```python
from build123d import *

# Parameters (mm, degrees)
SKETCH_1_R           = 3.1
EXTRUDE_1_DEPTH      = 6
SKETCH_2_R           = 3.1
CUT_EXTRUDE_6_DEPTH  = 2
SKETCH_4_R           = 1.5
CUT_EXTRUDE_7_DEPTH  = 118.034622889
CUT_EXTRUDE_8_REACH  = 119.12
SKETCH_5_W           = 7
SKETCH_5_H           = 21.556656584
SKETCH_5_W_2         = 5.195776916
SKETCH_5_R           = 4
SKETCH_5_W_3         = 8.137387099
SKETCH_5_H_2         = 20
SKETCH_5_W_4         = 10
SKETCH_6_R           = 3.1
CUT_EXTRUDE_9_DEPTH  = 2
SKETCH_7_R           = 1.6
CUT_EXTRUDE_10_DEPTH = 118.034622889
SKETCH_8_R           = 1.5
CUT_EXTRUDE_11_DEPTH = 118.120036521
SKETCH_9_W           = 120
SKETCH_9_H           = 5
CUT_EXTRUDE_12_DEPTH = 2
CHAMFER_1_SIZE       = 2
SKETCH_10_W          = 120
SKETCH_10_H          = 4
EXTRUDE_2_DEPTH      = 2


with BuildPart() as part:
    # 草图1 → 凸台-拉伸1 (new body)
    with BuildSketch(Plane.XY):
        with BuildLine():
            Line((53.211823486, 15.105307707), (98.846336292, -57.534028788))
            Line((98.846336292, -57.534028788), (98.846336292, -62.534028788))
            Line((98.846336292, -62.534028788), (-21.153663708, -62.534028788))
            Line((-21.153663708, -62.534028788), (-21.153663708, -57.534028788))
            Line((-21.153663708, -57.534028788), (18.804405563, 14.198660069))
            ThreePointArc((18.804405563, 14.198660069), (35.749695352, 24.459031414), (53.211823486, 15.105307707))
        make_face()
        with Locations((36.276519563, 4.465971212)):
            Circle(SKETCH_1_R, mode=Mode.SUBTRACT)
    extrude(amount=EXTRUDE_1_DEPTH)

    # 草图2 → 切除-拉伸6 (cut)
    with BuildSketch(Plane.XY.offset(6)):
        with Locations((29.276519563, 11.465971212)):
            Circle(SKETCH_2_R)
        with Locations(Location((43.276519563, 11.465971212, 0), (0, 0, 180))):
            Circle(SKETCH_2_R)
        with Locations((43.276519563, -2.534028788)):
            Circle(SKETCH_2_R)
        with Locations(Location((29.276519563, -2.534028788, 0), (0, 0, 180))):
            Circle(SKETCH_2_R)
    extrude(amount=-CUT_EXTRUDE_6_DEPTH, mode=Mode.SUBTRACT)

    # 草图4 → 切除-拉伸7 (cut, through all)
    with BuildSketch(Plane.XY.offset(4)):
        with Locations((43.276519563, 11.465971212)):
            Circle(SKETCH_4_R)
        with Locations((43.276519563, -2.534028788)):
            Circle(SKETCH_4_R)
        with Locations((29.276519563, -2.534028788)):
            Circle(SKETCH_4_R)
        with Locations((29.276519563, 11.465971212)):
            Circle(SKETCH_4_R)
    extrude(amount=-CUT_EXTRUDE_7_DEPTH, mode=Mode.SUBTRACT)

    # 草图5 → 切除-拉伸8 (cut, up to next)
    with BuildSketch(Plane.XY.offset(6), mode=Mode.PRIVATE) as cut_extrude_8_sk1:
        with Locations((21.160819148, -19.755700496)):
            Rectangle(SKETCH_5_W, SKETCH_5_H)
    cut_extrude_8_tool1 = extrude(cut_extrude_8_sk1.sketch, amount=-CUT_EXTRUDE_8_REACH, mode=Mode.PRIVATE) & part.part
    # 草图5 → 切除-拉伸8 (cut, up to next)
    with BuildSketch(Plane.XY.offset(6), mode=Mode.PRIVATE) as cut_extrude_8_sk2:
        with Locations((31.160819148, -19.755700496)):
            Rectangle(SKETCH_5_W, SKETCH_5_H)
    cut_extrude_8_tool2 = extrude(cut_extrude_8_sk2.sketch, amount=-CUT_EXTRUDE_8_REACH, mode=Mode.PRIVATE) & part.part
    # 草图5 → 切除-拉伸8 (cut, up to next)
    with BuildSketch(Plane.XY.offset(6), mode=Mode.PRIVATE) as cut_extrude_8_sk3:
        with Locations((41.160819148, -19.755700496)):
            Rectangle(SKETCH_5_W, SKETCH_5_H)
    cut_extrude_8_tool3 = extrude(cut_extrude_8_sk3.sketch, amount=-CUT_EXTRUDE_8_REACH, mode=Mode.PRIVATE) & part.part
    # 草图5 → 切除-拉伸8 (cut, up to next)
    with BuildSketch(Plane.XY.offset(6), mode=Mode.PRIVATE) as cut_extrude_8_sk4:
        with Locations((51.160819148, -19.755700496)):
            Rectangle(SKETCH_5_W, SKETCH_5_H)
    cut_extrude_8_tool4 = extrude(cut_extrude_8_sk4.sketch, amount=-CUT_EXTRUDE_8_REACH, mode=Mode.PRIVATE) & part.part
    # 草图5 → 切除-拉伸8 (cut, up to next)
    with BuildSketch(Plane.XY.offset(6), mode=Mode.PRIVATE) as cut_extrude_8_sk5:
        with Locations((60.258707606, -19.755700496)):
            Rectangle(SKETCH_5_W_2, SKETCH_5_H)
    cut_extrude_8_tool5 = extrude(cut_extrude_8_sk5.sketch, amount=-CUT_EXTRUDE_8_REACH, mode=Mode.PRIVATE) & part.part
    # 草图5 → 切除-拉伸8 (cut, up to next)
    with BuildSketch(Plane.XY.offset(6), mode=Mode.PRIVATE) as cut_extrude_8_sk6:
        with Locations((14.988200827, -44.534028788)):
            Circle(SKETCH_5_R)
    cut_extrude_8_tool6 = extrude(cut_extrude_8_sk6.sketch, amount=-CUT_EXTRUDE_8_REACH, mode=Mode.PRIVATE) & part.part
    # 草图5 → 切除-拉伸8 (cut, up to next)
    with BuildSketch(Plane.XY.offset(6), mode=Mode.PRIVATE) as cut_extrude_8_sk7:
        with Locations((44.988200827, -44.534028788)):
            Circle(SKETCH_5_R)
    cut_extrude_8_tool7 = extrude(cut_extrude_8_sk7.sketch, amount=-CUT_EXTRUDE_8_REACH, mode=Mode.PRIVATE) & part.part
    # 草图5 → 切除-拉伸8 (cut, up to next)
    with BuildSketch(Plane.XY.offset(6), mode=Mode.PRIVATE) as cut_extrude_8_sk8:
        with Locations((74.988200827, -44.534028788)):
            Circle(SKETCH_5_R)
    cut_extrude_8_tool8 = extrude(cut_extrude_8_sk8.sketch, amount=-CUT_EXTRUDE_8_REACH, mode=Mode.PRIVATE) & part.part
    # 草图5 → 切除-拉伸8 (cut, up to next)
    with BuildSketch(Plane.XY.offset(6), mode=Mode.PRIVATE) as cut_extrude_8_sk9:
        with Locations((1.433627507, -44.534028788)):
            Rectangle(SKETCH_5_W_3, SKETCH_5_H_2)
    cut_extrude_8_tool9 = extrude(cut_extrude_8_sk9.sketch, amount=-CUT_EXTRUDE_8_REACH, mode=Mode.PRIVATE) & part.part
    # 草图5 → 切除-拉伸8 (cut, up to next)
    with BuildSketch(Plane.XY.offset(6), mode=Mode.PRIVATE) as cut_extrude_8_sk10:
        with Locations((30.502321056, -44.534028788)):
            Rectangle(SKETCH_5_W_4, SKETCH_5_H_2)
    cut_extrude_8_tool10 = extrude(cut_extrude_8_sk10.sketch, amount=-CUT_EXTRUDE_8_REACH, mode=Mode.PRIVATE) & part.part
    # 草图5 → 切除-拉伸8 (cut, up to next)
    with BuildSketch(Plane.XY.offset(6), mode=Mode.PRIVATE) as cut_extrude_8_sk11:
        with Locations((60.502321056, -44.534028788)):
            Rectangle(SKETCH_5_W_4, SKETCH_5_H_2)
    cut_extrude_8_tool11 = extrude(cut_extrude_8_sk11.sketch, amount=-CUT_EXTRUDE_8_REACH, mode=Mode.PRIVATE) & part.part
    add(cut_extrude_8_tool1.solids().sort_by_distance((21.160819, -19.7557, 6))[0], mode=Mode.SUBTRACT)
    add(cut_extrude_8_tool2.solids().sort_by_distance((31.160819, -19.7557, 6))[0], mode=Mode.SUBTRACT)
    add(cut_extrude_8_tool3.solids().sort_by_distance((41.160819, -19.7557, 6))[0], mode=Mode.SUBTRACT)
    add(cut_extrude_8_tool4.solids().sort_by_distance((51.160819, -19.7557, 6))[0], mode=Mode.SUBTRACT)
    add(cut_extrude_8_tool5.solids().sort_by_distance((60.258708, -19.7557, 6))[0], mode=Mode.SUBTRACT)
    add(cut_extrude_8_tool6.solids().sort_by_distance((14.988201, -44.534029, 6))[0], mode=Mode.SUBTRACT)
    add(cut_extrude_8_tool7.solids().sort_by_distance((44.988201, -44.534029, 6))[0], mode=Mode.SUBTRACT)
    add(cut_extrude_8_tool8.solids().sort_by_distance((74.988201, -44.534029, 6))[0], mode=Mode.SUBTRACT)
    add(cut_extrude_8_tool9.solids().sort_by_distance((1.433628, -44.534029, 6))[0], mode=Mode.SUBTRACT)
    add(cut_extrude_8_tool10.solids().sort_by_distance((30.502321, -44.534029, 6))[0], mode=Mode.SUBTRACT)
    add(cut_extrude_8_tool11.solids().sort_by_distance((60.502321, -44.534029, 6))[0], mode=Mode.SUBTRACT)

    # 草图6 → 切除-拉伸9 (cut)
    with BuildSketch(Plane.XY.offset(6)):
        with Locations((21.502321056, -37.534028788)):
            Circle(SKETCH_6_R)
        with Locations((9.502321056, -37.534028788)):
            Circle(SKETCH_6_R)
        with Locations((9.502321056, -51.534028788)):
            Circle(SKETCH_6_R)
        with Locations((21.502321056, -51.534028788)):
            Circle(SKETCH_6_R)
        with Locations((39.502321056, -37.534028788)):
            Circle(SKETCH_6_R)
        with Locations((51.502321056, -37.534028788)):
            Circle(SKETCH_6_R)
        with Locations((51.502321056, -51.534028788)):
            Circle(SKETCH_6_R)
        with Locations((39.502321056, -51.534028788)):
            Circle(SKETCH_6_R)
        with Locations((69.502321056, -37.534028788)):
            Circle(SKETCH_6_R)
        with Locations((81.502321056, -37.534028788)):
            Circle(SKETCH_6_R)
        with Locations((81.502321056, -51.534028788)):
            Circle(SKETCH_6_R)
        with Locations((69.502321056, -51.534028788)):
            Circle(SKETCH_6_R)
    extrude(amount=-CUT_EXTRUDE_9_DEPTH, mode=Mode.SUBTRACT)

    # 草图7 → 切除-拉伸10 (cut, through all)
    with BuildSketch(Plane.XY.offset(4)):
        with Locations((9.502321056, -37.534028788)):
            Circle(SKETCH_7_R)
        with Locations((21.502321056, -37.534028788)):
            Circle(SKETCH_7_R)
        with Locations((9.502321056, -51.534028788)):
            Circle(SKETCH_7_R)
        with Locations((21.502321056, -51.534028788)):
            Circle(SKETCH_7_R)
        with Locations((51.502321056, -51.534028788)):
            Circle(SKETCH_7_R)
        with Locations((39.502321056, -51.534028788)):
            Circle(SKETCH_7_R)
        with Locations((39.502321056, -37.534028788)):
            Circle(SKETCH_7_R)
        with Locations((51.502321056, -37.534028788)):
            Circle(SKETCH_7_R)
        with Locations((81.502321056, -51.534028788)):
            Circle(SKETCH_7_R)
        with Locations((69.502321056, -51.534028788)):
            Circle(SKETCH_7_R)
        with Locations((69.502321056, -37.534028788)):
            Circle(SKETCH_7_R)
        with Locations((81.502321056, -37.534028788)):
            Circle(SKETCH_7_R)
    extrude(amount=-CUT_EXTRUDE_10_DEPTH, mode=Mode.SUBTRACT)

    # 草图8 → 切除-拉伸11 (cut, through all)
    with BuildSketch(Plane.XY.offset(6)):
        with Locations((90.502321056, -60.034028788)):
            Circle(SKETCH_8_R)
        with Locations((60.502321056, -60.034028788)):
            Circle(SKETCH_8_R)
        with Locations((30.502321056, -60.034028788)):
            Circle(SKETCH_8_R)
        with Locations((0.502321056, -60.034028788)):
            Circle(SKETCH_8_R)
        with Locations((-14.497678944, -60.034028788)):
            Circle(SKETCH_8_R)
    extrude(amount=-CUT_EXTRUDE_11_DEPTH, mode=Mode.SUBTRACT)

    # 草图9 → 切除-拉伸12 (cut)
    with BuildSketch(Plane.XY.offset(6)):
        with Locations((38.846336292, -60.034028788)):
            Rectangle(SKETCH_9_W, SKETCH_9_H)
    extrude(amount=-CUT_EXTRUDE_12_DEPTH, mode=Mode.SUBTRACT)

    # 倒角1
    chamfer_1_edges = [part.edges().sort_by_distance(p)[0] for p in [
        (38.846336292, -57.534028788, 6),
    ]]
    chamfer(chamfer_1_edges, length=CHAMFER_1_SIZE - 0.0001)  # a hair under: the kernel refuses the full size

    # 草图10 → 凸台-拉伸2 (add)
    with BuildSketch(Plane.XZ.offset(62.534028788)):
        with Locations((38.846336292, 2)):
            Rectangle(SKETCH_10_W, SKETCH_10_H)
    extrude(amount=EXTRUDE_2_DEPTH)


solid = part.part
```
Input: part model. Units: mm. Frame: model coordinates. A direction names the side the tool comes from. Coordinates: 2 decimals unless noted, no trailing zeros. Loops run counter-clockwise (first coordinate to the right, second up) from the corner with the lowest first, then second, coordinate; pieces in that order, holes last.
Q1. Section B-B, the plane x = 21.5. Give the number of separate pieces and of enclosed holes in the cut face, and give its area (3 significant figures).
Results are:
separate pieces: 4
enclosed holes: 0
area: 299 mm2
Q2. Section A-A, the plane y = -16. Return the cut outline in (x, z).
Results are:
outline: (1.98, 0) - (17.66, 0) - (17.66, 6) - (1.98, 6) - close; (24.66, 0) - (27.66, 0) - (27.66, 6) - (24.66, 6) - close; (34.66, 0) - (37.66, 0) - (37.66, 6) - (34.66, 6) - close; (44.66, 0) - (47.66, 0) - (47.66, 6) - (44.66, 6) - close; (54.66, 0) - (57.66, 0) - (57.66, 6) - (54.66, 6) - close; (62.86, 0) - (72.75, 0) - (72.75, 6) - (62.86, 6) - close
Q3. Set-up query: faces 1 (the flat face through (31, -8.977, 3)), 2 (the cylindrical face through (54.366, -38.721, 5.014)). Return all of +Z, -Z, +X, -X, +Y, -Y with unobstructed straight access to the full face (end or side cutting, diameter ignored); none if empty.
Results are:
face 1: +Z, -Z
face 2: +Z
Q4. Line query: line 1 along Y through (x, z) = (81.5, 1); line 2 along Y through (x, z) = (82.5, 3.5); line 3 along Y through (x, z) = (61, 3.25). Output: solid intervals per line, ascending.
Results are:
line 1: y = -64.53 to -53.13, -49.93 to -39.13, -35.93 to -29.92
line 2: y = -64.53 to -52.78, -50.28 to -38.78, -36.28 to -31.51
line 3: y = -64.53 to -61.45, -58.62 to -54.53, -34.53 to -30.53, -8.98 to 2.71
Q5. Contact query for flat-ended pins moving along their axis: pin 1 (2 mm diameter, centred on y = 10, z = 2, fed in from -X); pin 2 (3 mm diameter, centred on x = 40, z = 2.5, fed in from +Y); pin 3 (3.5 mm diameter, centred on x = 21.5, y = -37.53, fed in from +Z). Output: stop coordinate, or through.
Results are:
pin 1: stops at x = 15.91
pin 2: stops at y = 24.34
pin 3: stops at z = 4
